Here's the drawing with two shaded views (mm, measured from the low corner). I have some questions. A direction names the side the tool comes from. Give positions to 0.01 mm unless a question says otherwise; leave off trailing zeros. Loops run counter-clockwise (first coordinate to the right, second up) from the corner with the lowest first, then second, coordinate; pieces in that order, holes last.
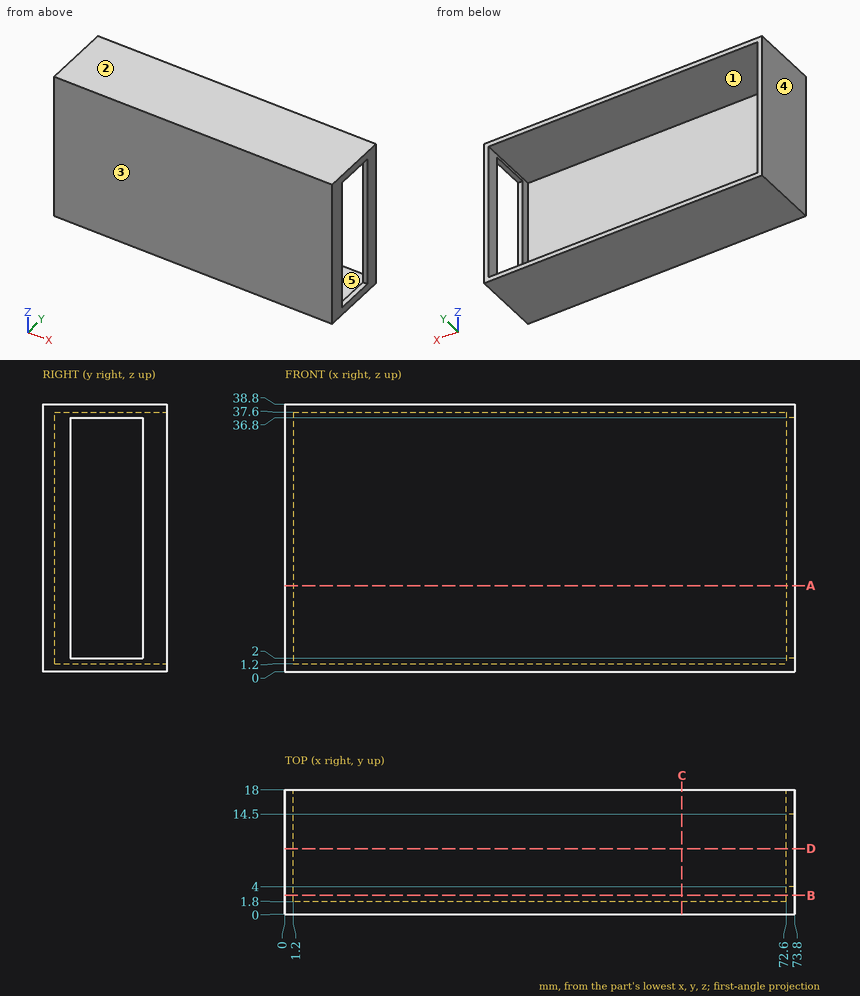
(1) Suppose I cut it at B-B on y = 2.75. List the corners of the cut face in (x, z) for me.
Returned:
outline: (0, 0) - (73.8, 0) - (73.8, 38.8) - (0, 38.8) - close; hole (1.2, 1.2) - (72.6, 1.2) - (72.6, 37.6) - (1.2, 37.6) - close
(2) Suppose I cut it at C-C on x = 57.5. List the corners of the cut face in (y, z) for me, plus the area to 3 significant figures.
Returned:
outline: (0, 0) - (18, 0) - (18, 1.2) - (1.8, 1.2) - (1.8, 37.6) - (18, 37.6) - (18, 38.8) - (0, 38.8) - close
area: 109 mm2
(3) Suppose I cut it at A-A on z = 12.5. List the corners of the cut face in (x, y) for me.
Returned:
outline: (0, 0) - (73.8, 0) - (73.8, 4) - (72.6, 4) - (72.6, 1.8) - (1.2, 1.8) - (1.2, 18) - (0, 18) - close; (72.6, 14.5) - (73.8, 14.5) - (73.8, 18) - (72.6, 18) - close
(4) Suppose I cut it at D-D on y = 9.5. List the corners of the cut face in (x, z) for me.
Returned:
outline: (0, 0) - (73.8, 0) - (73.8, 2) - (72.6, 2) - (72.6, 1.2) - (1.2, 1.2) - (1.2, 37.6) - (72.6, 37.6) - (72.6, 36.8) - (73.8, 36.8) - (73.8, 38.8) - (0, 38.8) - close
(5) Please list where these lines run through material, in increasing order: probe 1 along Z at (x, y) = (19, 11.5); probe 2 along X at (y, z) = (3.5, 16); probe 3 along Y at (x, z) = (16.5, 9).
Returned:
probe 1: z = 0 to 1.2, 37.6 to 38.8
probe 2: x = 0 to 1.2, 72.6 to 73.8
probe 3: y = 0 to 1.8
(6) Thinking about a two-plate mould opening in Z: for the marked faces 1, 2 and 3, which applies, pulls with the +Z half, pulls with the -Z half, needs draft (parallel to the pull), parting line crosses it, or undercut?
Returned:
face 1: undercut
face 2: pulls with the +Z half
face 3: needs draft
(7) Will this pin go through, and if not, where does the flat tip stop? P1, Ø10, axis at x = 9, z = 31.5, coming from the +Y side.
Returned:
P1: stops at y = 1.8
(8) Which directions (+Z, -Z, +X, -X, +Y, -Y) give clear straight access to the entire face, cutting with the end or side of a thin tool? Please do the marked faces 4 and 5.
Returned:
face 4: +Z, -Z, -X, +Y, -Y
face 5: +Y
